Part print with two shaded views. Sizes in mm from the minimum x, y, z corner. A direction names the side the tool comes from. Give positions to 0.01 mm unless a question says otherwise; leave off trailing zeros. Order: outer loops, then holes, each group sorted by start corner. A loop starts at its lowest first (then second) coordinate and runs counter-clockwise, first axis right, second up. Notation, with made-up numbers: M 56,69 L 111,69 A9 ccw 111,76 Z; hole C 8,32 d10. An arc over 180 degrees is marked long. Write each question's results on one line, items separated by ' | '. Start each with the question number.
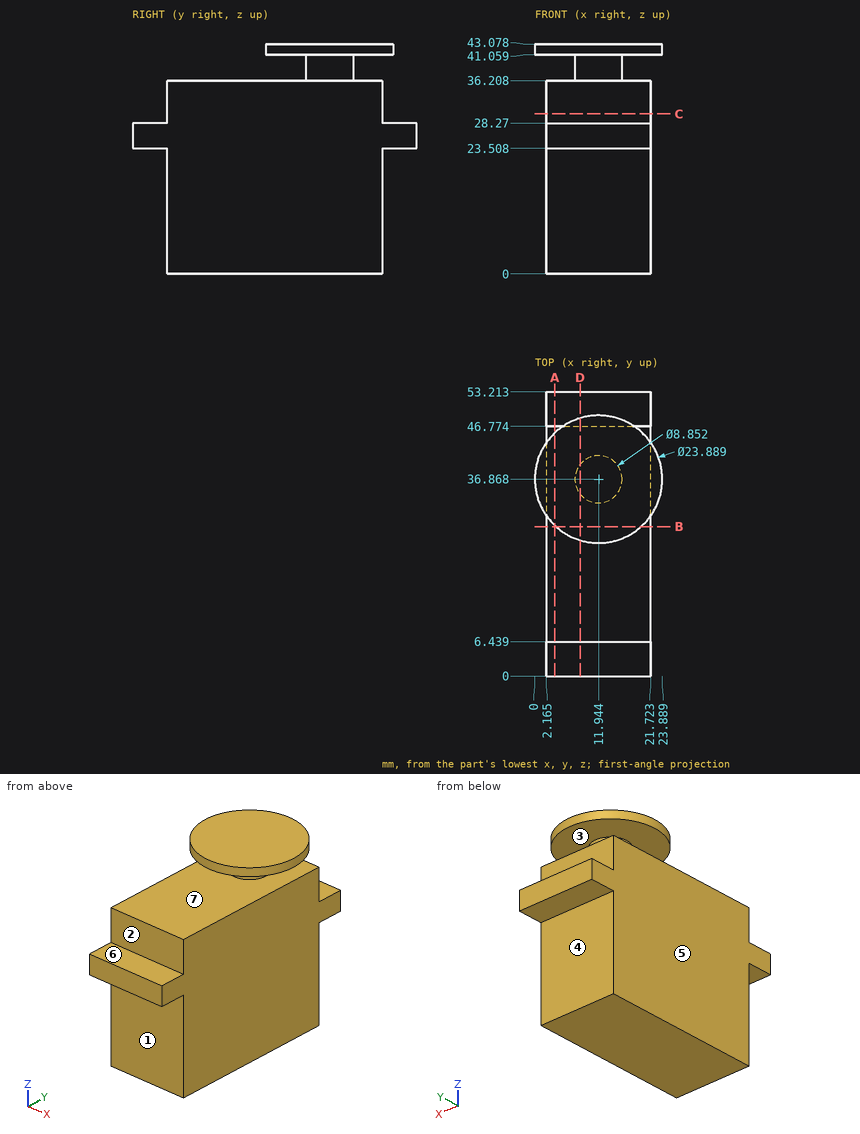
(1) Probe L1, parallel to Z at x = 12, y = 30.5; L2, parallel to Y at x = 18.75, z = 6.5; L3, parallel to X at y = 30.5, z = 10 (1 decimal). List the from-to ranges inside material, lowest first.
(2) Saw through at D-D on x = 8.5. Give the cut face in (y, z) (1 decimal), plus the area to 4 significant figures.
(3) Tool access for the marked faces 1, 2, 3 and 4: list every direction of +Z, -Z, +X, -X, +Y, -Y with a clear straight run to the whole face (end or side of a thin tool).
(4) Pull direction Z, two halves, no side cores. Call the marked faces 5, 6 and 7: +Z half, -Z half, draft (parallel to the pull), parting line (faces both ways), or undercut.
(5) Saw through at C-C on z = 30. Give the cut face in (x, y) (1 decimal).
(6) Saw through at A-A on x = 3.75. Give the cut face in (y, z).
(7) Drop flat-ended pins along their axis: P1, Ø6, axis at x = 10.5, z = 35, coming from the -Y side; P2, Ø12, axis at x = 16, y = 31.5, coming from the -Z side; P3, Ø12, axis at x = 20.5, y = 17, coming from the +Z side; P4, Ø1.5, axis at y = 45.5, z = 6, coming from the +X side. Give the stop position or say it passes through.
(8) Saw through at B-B on y = 28. Give the cut face in (x, z) (1 decimal).
Taken from the geometry:
1) L1: z = 0 to 36.21, 41.06 to 43.08 | L2: y = 6.44 to 46.77 | L3: x = 2.2 to 21.7
2) outline: M 0,23.5 L 6.4,23.5 L 6.4,0 L 46.8,0 L 46.8,23.5 L 53.2,23.5 L 53.2,28.3 L 46.8,28.3 L 46.8,36.2 L 39.6,36.2 L 39.6,41.1 L 48.3,41.1 L 48.3,43.1 L 25.4,43.1 L 25.4,41.1 L 34.1,41.1 L 34.1,36.2 L 6.4,36.2 L 6.4,28.3 L 0,28.3 Z | area: 1,595 mm²
3) face 1: -Z, +X, -X, -Y | face 2: +Z, +X, -X, -Y | face 3: none | face 4: -Z, +X, -X, +Y
4) face 5: draft | face 6: +Z half | face 7: undercut
5) outline: M 2.2,6.4 L 21.7,6.4 L 21.7,46.8 L 2.2,46.8 Z
6) outline: M 0,23.51 L 6.44,23.51 L 6.44,0 L 46.77,0 L 46.77,23.51 L 53.21,23.51 L 53.21,28.27 L 46.77,28.27 L 46.77,36.21 L 6.44,36.21 L 6.44,28.27 L 0,28.27 Z; M 28.18,41.06 L 45.56,41.06 L 45.56,43.08 L 28.18,43.08 Z
7) P1: stops at y = 6.44 | P2: stops at z = 0 | P3: stops at z = 36.21 | P4: stops at x = 21.72
8) outline: M 2.2,0 L 21.7,0 L 21.7,36.2 L 2.2,36.2 Z; M 3.9,41.1 L 19.9,41.1 L 19.9,43.1 L 3.9,43.1 Z
